Source: CAD feature listing. Evaluate the final solid. Frame: model axes, mm. Give positions to 0.01 mm unless a question says otherwise; leave off trailing zeros. Write each loop counter-clockwise with the first axis right and the second up, starting at its lowest first coordinate (ties: lowest second). Pieces come first, ordered by that corner, then holes. Notation, with made-up numbers: (69.5, -31) -> (90.5, -31) arc R23 cw to (90.5, -3) -> close; hole circle Ø10 at (61, 18.25). An arc over 180 degrees is marked (long way). Write item = value, one per line.
from build123d import *

# Parameters (mm, degrees)
BOSS_EXTRUDE1_DEPTH = 3.175


with BuildPart() as part:
    # Sketch1 → Boss-Extrude1 (new body)
    with BuildSketch(Plane.XY):
        Polygon((-228.7016, 8.62965), (-203.3016, 8.62965), (-203.3016, 5.65785), (-228.7016, 5.65785), (-228.7016, -5.65785), (-203.3016, -5.65785), (-203.3016, -8.62965), (-228.7016, -8.62965), (-228.7016, -55.273575), (222.1484, -55.273575), (222.1484, -61.547375), (-228.7016, -61.547375), (-228.7016, -72.4662), (228.7016, -72.4662), (228.7016, -8.62965), (203.3016, -8.62965), (203.3016, -5.65785), (228.7016, -5.65785), (228.7016, 5.65785), (203.3016, 5.65785), (203.3016, 8.62965), (228.7016, 8.62965), (228.7016, 72.4662), (-228.7016, 72.4662), (-228.7016, 61.547375), (222.1484, 61.547375), (222.1484, 55.273575), (-228.7016, 55.273575), align=None)
        Polygon((222.1484, -48.720375), (222.1484, -15.9766), (196.7484, -15.9766), (196.7484, 15.9766), (222.1484, 15.9766), (222.1484, 48.720375), (-222.1484, 48.720375), (-222.1484, 15.9766), (-196.7484, 15.9766), (-196.7484, -15.9766), (-222.1484, -15.9766), (-222.1484, -48.720375), align=None, mode=Mode.SUBTRACT)
    extrude(amount=BOSS_EXTRUDE1_DEPTH)


solid = part.part
(1) Material intervals for line 1 (Y direction, x = -103.5, z = 1.55); line 2 (X direction, y = 42.5, z = 1.3); line 3 (X direction, y = 6, z = 2.1), sorted ascending.
Values follow:
line_1 = -72.47 to -61.55, -55.27 to -48.72, 48.72 to 55.27, 61.55 to 72.47
line_2 = -228.7 to -222.15, 222.15 to 228.7
line_3 = -203.3 to -196.75, 196.75 to 203.3
(2) Section query A-A (y = 43.5). Return loops of the section in (x, z) (3 decimals), plus the area to 3 significant figures.
Values follow:
outline = (-228.702, 0) -> (-222.148, 0) -> (-222.148, 3.175) -> (-228.702, 3.175) -> close; (222.148, 0) -> (228.702, 0) -> (228.702, 3.175) -> (222.148, 3.175) -> close
area = 41.6 mm2
(3) First-contact query: pin 1 (0.9 mm diameter, centred on y = -8, z = 1.5, fed in from -X); pin 2 (0.9 mm diameter, centred on y = 7, z = 2, fed in from +X). Flat tips, straight axial feed; report the tip coordinate or a pass-through.
Values follow:
pin_1 = -203.3
pin_2 = 203.3
(4) Section query B-B (x = -9). Return loops of the section in (y, z) (3 decimals).
Values follow:
outline = (-72.466, 0) -> (-61.547, 0) -> (-61.547, 3.175) -> (-72.466, 3.175) -> close; (-55.274, 0) -> (-48.72, 0) -> (-48.72, 3.175) -> (-55.274, 3.175) -> close; (48.72, 0) -> (55.274, 0) -> (55.274, 3.175) -> (48.72, 3.175) -> close; (61.547, 0) -> (72.466, 0) -> (72.466, 3.175) -> (61.547, 3.175) -> close
